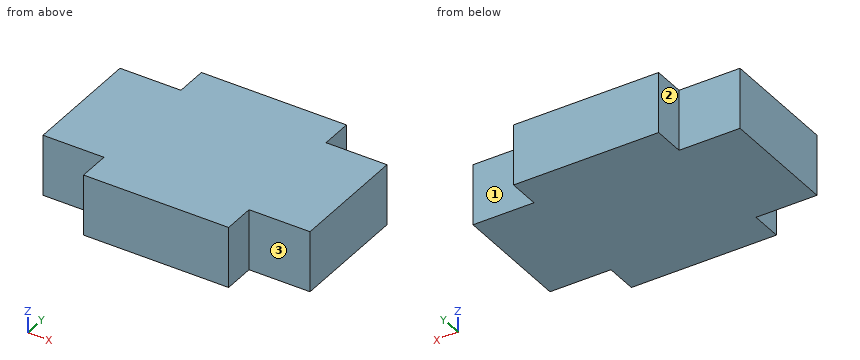
from build123d import *

# Parameters (mm, degrees)
F0_W     = 5
F0_H     = 9.8
F1_DEPTH = 5


with BuildPart() as f1:
    # F0 (on Top) → F1 (new body)
    with BuildSketch(Plane.XY):
        Polygon((-5.95, -4.9), (-5.95, 4.9), (-10.95, 4.9), (-10.95, 0), (-10.95, -4.9), align=None)
        Polygon((5.95, 4.9), (5.95, 7.5), (-5.95, 7.5), (-5.95, 4.9), (-5.95, -4.9), (-5.95, -7.5), (5.95, -7.5), (5.95, -4.9), align=None)
        with Locations((8.45, 0)):
            Rectangle(F0_W, F0_H)
    extrude(amount=F1_DEPTH)


solid = f1.part
Here's how the part is built. I have some questions about the finished solid (model axes, mm). Face numbers are marked on the shaded views. A direction names the side the tool comes from. Give positions to 0.01 mm unless a question says otherwise; leave off trailing zeros. Loops run counter-clockwise (first coordinate to the right, second up) from the corner with the lowest first, then second, coordinate; pieces in that order, holes last. Notation, with made-up numbers: (30, 58.5) -> (63, 58.5) arc R23 cw to (63, 83.5) -> close; hole circle Ø3 at (3.5, 41.25). An arc over 180 degrees is marked (long way). Answer as a JSON object with one key per item and string values. Group by question number.
Item 1: On a 3-axis mill with a long thin cutter (end or side, diameter ignored), from which of +Z, -Z, +X, -X, +Y, -Y can I reach the whole of each face in a straight line? I mean the marked faces 1, 2 and 3. Say none if no direction works.
Item 2: I need wall thicknesses on L1, parallel to X at y = 5.5, z = 2.6; L2, parallel to Y at x = 8.75, z = 3.65. Which ranges of each line are inside material? Lowest first, please.
Item 3: Imagine slicing it at A-A on z = 1. Write out the boundary of the cut face in (x, y), then the cut area to 4 significant figures.
Item 4: Imagine slicing it at B-B on y = 6.75. Write out the boundary of the cut face in (x, z), then the cut area to 3 significant figures.
Item 5: Imagine slicing it at C-C on x = -9.5. Write out the boundary of the cut face in (y, z), then the cut area to 3 significant figures.
Item 6: Will these pins go through, and if not, where does the flat tip stop? pin 1 (1.5 mm diameter, centred on x = -7.5, z = 3, fed in from -Y); pin 2 (3 mm diameter, centred on y = 7, z = 3.5, fed in from -X); pin 3 (0.8 mm diameter, centred on y = -6.5, z = 1.5, fed in from +X).
Answer list:
{
 "1": {"face 1": "+Z, -Z, +X, +Y", "face 2": "+Z, -Z, -X, +Y", "face 3": "+Z, -Z, +X, -Y"},
 "2": {"L1": "x = -5.95 to 5.95", "L2": "y = -4.9 to 4.9"},
 "3": {"outline": "(-10.95, -4.9) -> (-5.95, -4.9) -> (-5.95, -7.5) -> (5.95, -7.5) -> (5.95, -4.9) -> (10.95, -4.9) -> (10.95, 4.9) -> (5.95, 4.9) -> (5.95, 7.5) -> (-5.95, 7.5) -> (-5.95, 4.9) -> (-10.95, 4.9) -> close", "area": "276.5 mm2"},
 "4": {"outline": "(-5.95, 0) -> (5.95, 0) -> (5.95, 5) -> (-5.95, 5) -> close", "area": "59.5 mm2"},
 "5": {"outline": "(-4.9, 0) -> (4.9, 0) -> (4.9, 5) -> (-4.9, 5) -> close", "area": "49.0 mm2"},
 "6": {"pin 1": "stops at y = -4.9", "pin 2": "stops at x = -5.95", "pin 3": "stops at x = 5.95"}
}
